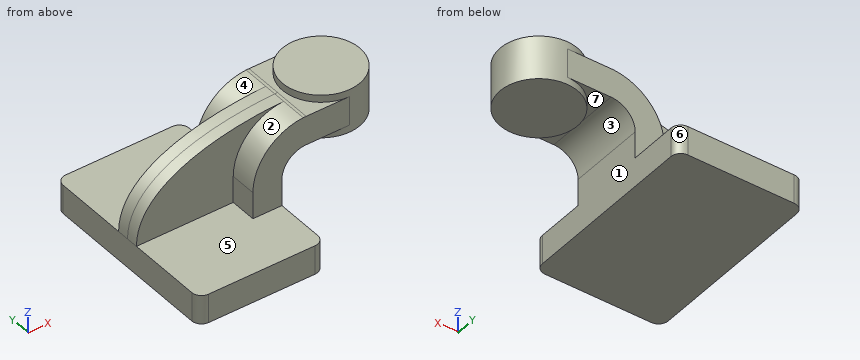
from build123d import *

# Parameters (mm, degrees)
F1_DEPTH = 63.5
F2_DEPTH = 25.4
F3_DEPTH = 7.9375
F5_R     = 6.35


with BuildPart() as f1:
    # F0 (on Front) → F1 (new body, symmetric)
    with BuildSketch(Plane.XZ):
        Polygon((-41.275, 9.525), (-41.275, -9.525), (41.275, -9.525), (41.275, 9.525), (22.225, 9.525), align=None)
    extrude(amount=F1_DEPTH, both=True)

    # F0 (on Front) → F2 (join, symmetric)
    with BuildSketch(Plane.XZ):
        with BuildLine():
            Line((22.225, 9.525), (41.275, 9.525))
            Line((41.275, 9.525), (41.275, 27.0002))
            ThreePointArc((41.275, 27.0002), (45.9246798487, 38.2255201513), (57.15, 42.8752))
            Line((57.15, 42.8752), (60.325, 42.8752))
            Line((60.325, 42.8752), (60.325, 61.9252))
            Line((60.325, 61.9252), (57.15, 61.9252))
            add(Edge.make_bspline(
                [(55.2851476574, 61.8753767127), (55.9059880343, 61.8941041264), (56.5276296664, 61.9107089301), (57.15, 61.9252)],
                knots=[110.161512309, 110.161512309, 110.161512309, 110.161512309, 111.5045361635, 111.5045361635, 111.5045361635, 111.5045361635], degree=3))
            ThreePointArc((55.2851476574, 61.8753767127), (31.8035446949, 51.0275350263), (22.225, 27.0002))
            Line((22.225, 27.0002), (22.225, 9.525))
        make_face()
        Polygon((75.3291722601, 61.9252), (60.325, 61.9252), (60.325, 42.8752), (75.3291722601, 42.8752), (85.725, 42.8752), (85.725, 61.9252), align=None)
    extrude(amount=F2_DEPTH, both=True)

    # F0 (on Front) → F3 (join, symmetric)
    with BuildSketch(Plane.XZ):
        with BuildLine():
            add(Edge.make_bspline(
                [(-41.275, 9.525), (-41.1727746696, 44.5220155957), (4.3607246911, 60.3392608693), (55.2851476574, 61.8753767127)],
                knots=[0, 0, 0, 0, 110.161512309, 110.161512309, 110.161512309, 110.161512309], degree=3))
            Line((-41.275, 9.525), (22.225, 9.525))
            Line((22.225, 9.525), (22.225, 27.0002))
            ThreePointArc((22.225, 27.0002), (31.8035446949, 51.0275350263), (55.2851476574, 61.8753767127))
        make_face()
    extrude(amount=F3_DEPTH, both=True)

    # F0 (on Front) → F4 (revolve)
    with BuildSketch(Plane.XZ):
        Polygon((111.125, 66.675), (85.725, 66.675), (85.725, 61.9252), (85.725, 42.8752), (85.725, 38.1), (111.125, 38.1), align=None)
    revolve(axis=Axis((85.725, 0, 52.3875), (0, 0, 1)))

    # F5
    f5_edges = [f1.edges().sort_by_distance(p)[0] for p in [
        (41.275, -63.5, 0),
        (-41.275, -63.5, 0),
        (41.275, 63.5, 0),
        (-41.275, 63.5, 0),
    ]]
    fillet(f5_edges, radius=F5_R)


solid = f1.part
For this review, take the finished solid that the model builds, in its own axes (mm). Face numbers are marked on the shaded views. A direction names the side the tool comes from. Give positions to 0.01 mm unless a question says otherwise; leave off trailing zeros. Loops run counter-clockwise (first coordinate to the right, second up) from the corner with the lowest first, then second, coordinate; pieces in that order, holes last. Notation, with made-up numbers: M -22,66.25 L 24,66.25 A27 ccw 24,102.25 Z; hole C 46.5,39.25 d9. An arc over 180 degrees is marked long. Put each result on its own line as item: value. Start each with the question number.
(1) Machinability: for the marked faces 1, 2, 3 and 4, which of the approach directions +Z, -Z, +X, -X, +Y, -Y give a long, thin tool a straight path to every point of the face, cutting with its end or side? Answer none if there is none.
(2) Add section C-C, the plane y = -52.5. Write out the cut boundary in (x, z) (3 decimals), then the cut area to 3 significant figures.
(3) Add section A-A, the plane z = -2. Write out the cut boundary in (x, y) (3 decimals).
(4) The part is to be moulded in two halves that separate along X. For the marked faces 5, 6 and 7, say which applies: +X half, -X half, draft (parallel to the pull), parting line (faces both ways), or undercut.
(5) Wall thickness on L1, parallel to X at y = 50, z = 1 (3 decimals); L2, parallel to X at y = -15.5, z = 13 (3 decimals); L3, parallel to Y at x = 63, z = 59.5: over which ranges is each line inside the solid? List them lowest first.
(6) For pin 1 (8.5 mm diameter, centred on x = 64.5, y = 6.5, fed in from -Z); pin 2 (8.5 mm diameter, centred on y = 16, z = 18.5, fed in from -X) (3 decimals); pin 3 (2 mm diameter, centred on x = 95, z = 37, fed in from +Y); pin 4 (8 mm diameter, centred on x = 26, y = 27.5, fed in from +Z), all flat-tipped, find the tip position at first contact; note any pin that passes through.
(7) Add section B-B, the plane x = 80. Write out the cut boundary in (y, z) (3 decimals).
Result:
1. face 1: -Z, +X, +Y, -Y
1. face 2: +Z, -X, -Y
1. face 3: -Z, +Y, -Y
1. face 4: +Z, -X, +Y
2. outline: M -41.275,-9.525 L 41.275,-9.525 L 41.275,9.525 L -41.275,9.525 Z
2. area: 1,570 mm^2
3. outline: M -41.275,-57.15 A6.35 ccw -34.925,-63.5 L 34.925,-63.5 A6.35 ccw 41.275,-57.15 L 41.275,57.15 A6.35 ccw 34.925,63.5 L -34.925,63.5 A6.35 ccw -41.275,57.15 Z
4. face 5: draft
4. face 6: +X half
4. face 7: undercut
5. L1: x = -41.275 to 41.275
5. L2: x = 22.225 to 41.275
5. L3: y = -25.4 to 25.4
6. pin 1: stops at z = 38.1
6. pin 2: stops at x = 22.225
6. pin 3: passes through
6. pin 4: stops at z = 48.21
7. outline: M -25.4,42.875 L -24.746,42.875 L -24.746,38.1 L 24.746,38.1 L 24.746,42.875 L 25.4,42.875 L 25.4,61.925 L 24.746,61.925 L 24.746,66.675 L -24.746,66.675 L -24.746,61.925 L -25.4,61.925 Z
